```python
from build123d import *

# Parameters (mm, degrees)
F0_R           = 13.5
F0_R_2         = 10.75
F1_DEPTH       = 5
F2_R           = 25
F2_R_2         = 13.5
F2_R_3         = 10.75
F3_DEPTH       = 7
F4_R           = 17.5
F5_DEPTH       = 27
F6_R           = 30
F6_R_2         = 17.5
F7_DEPTH       = 11
F8_R           = 22.5
F9_DEPTH       = 49
F10_R          = 15
F11_DEPTH      = 4
F12_R          = 17
F12_R_2        = 15
F13_DEPTH      = 5
F14_R          = 11.5
F15_DEPTH      = 37
F16_R          = 10.75
F17_DEPTH      = 103.001
F18_SIZE       = 0.5
F19_SIZE2      = 2.99999
F19_SIZE       = 7.49999
F20_SIZE       = 0.5
F22_R          = 10
F23_DEPTH      = 57
F23_DEPTH_BACK = 11
F24_R          = 8
F25_DEPTH      = 71.2396442793
F26_R          = 17
F26_R_2        = 10
F26_R_3        = 8
F27_DEPTH      = 7
F28_SIZE2      = 6.99999
F28_SIZE       = 2.99999
F30_R          = 1.25
F33_R          = 11.5
F34_DEPTH      = 1.1


# Not quite as in the source:
# - a fillet or chamfer that OpenCascade refuses, or shapes differently, is made with other operations: its cross-section is extruded or revolved along the edge and cut away or added
# - a fillet or chamfer is up to 0.001 mm smaller than in the source, because OpenCascade refuses the exact size


with BuildPart() as f1:
    # F0 (on Top) → F1 (new body)
    with BuildSketch(Plane.XY):
        Circle(F0_R)
        Circle(F0_R_2, mode=Mode.SUBTRACT)
    extrude(amount=F1_DEPTH)

    # F2 (on face) → F3 (join)
    with BuildSketch(Plane(origin=(0, 0, 0), x_dir=(1, 0, 0), z_dir=(0, 0, -1))):
        Circle(F2_R)
        Circle(F2_R_2, mode=Mode.SUBTRACT)
        Circle(F2_R_2)
        Circle(F2_R_3, mode=Mode.SUBTRACT)
    extrude(amount=F3_DEPTH)

    # F4 (on face) → F5 (join)
    with BuildSketch(Plane(origin=(0, 0, -7), x_dir=(1, 0, 0), z_dir=(0, 0, -1))):
        Circle(F4_R)
    extrude(amount=F5_DEPTH)

    # F6 (on face) → F7 (join)
    with BuildSketch(Plane(origin=(0, 0, -34), x_dir=(1, 0, 0), z_dir=(0, 0, -1))):
        Circle(F6_R)
        Circle(F6_R_2, mode=Mode.SUBTRACT)
        Circle(F6_R_2)
    extrude(amount=F7_DEPTH)

    # F8 (on face) → F9 (join)
    with BuildSketch(Plane(origin=(0, 0, -45), x_dir=(1, 0, 0), z_dir=(0, 0, -1))):
        Circle(F8_R)
    extrude(amount=F9_DEPTH)

    # F10 (on face) → F11 (join)
    with BuildSketch(Plane(origin=(0, 0, -94), x_dir=(1, 0, 0), z_dir=(0, 0, -1))):
        Circle(F10_R)
    extrude(amount=F11_DEPTH)

    # F12 (on face) → F13 (join)
    with BuildSketch(Plane(origin=(0, 0, -98), x_dir=(1, 0, 0), z_dir=(0, 0, -1))):
        Circle(F12_R)
        Circle(F12_R_2, mode=Mode.SUBTRACT)
        Circle(F12_R_2)
    extrude(amount=F13_DEPTH)

    # F14 (on face) → F15 (cut)
    with BuildSketch(Plane(origin=(0, 0, -103), x_dir=(1, 0, 0), z_dir=(0, 0, -1))):
        Circle(F14_R)
    extrude(amount=-F15_DEPTH, mode=Mode.SUBTRACT)

    # F16 (on face) → F17 (cut, through all)
    with BuildSketch(Plane.XY):
        Circle(F16_R)
    extrude(amount=-F17_DEPTH, mode=Mode.SUBTRACT)

    # F18
    f18_edges = [f1.edges().sort_by_distance(p)[0] for p in [
        (-11.5, 0, -103),
        (-22.5, 0, -94),
        (-30, 0, -45),
        (-30, 0, -34),
        (-25, 0, 0),
        (-13.5, 0, 5),
        (-10.75, 0, 5),
    ]]
    chamfer(f18_edges, length=F18_SIZE)

    # F19 (size 7.5 and 3 in the source; OpenCascade refuses exactly that, so slightly less here)
    f19_edges = [f1.edges().sort_by_distance(p)[0] for p in [
        (-25, 0, -7),
    ]]
    f19_side = f1.faces().sort_by_distance((-24.292893, 0, -7))[0]
    chamfer(f19_edges, length=F19_SIZE, length2=F19_SIZE2, reference=f19_side)

    # F20
    f20_edges = [f1.edges().sort_by_distance(p)[0] for p in [
        (-25, 0, -4.00001),
    ]]
    chamfer(f20_edges, length=F20_SIZE)

    # F22 (on offset) → F23 (join, two sides)
    with BuildSketch(Plane.XZ.offset(22.5)) as f23_sk:
        with Locations((0, -79)):
            Circle(F22_R)
    extrude(amount=F23_DEPTH)
    extrude(f23_sk.sketch, amount=-F23_DEPTH_BACK)

    # F24 (on face) → F25 (cut, through all)
    with BuildSketch(Plane.XZ.offset(79.5)):
        with Locations((0, -79)):
            Circle(F24_R)
    extrude(amount=-F25_DEPTH, mode=Mode.SUBTRACT)

    # F26 (on face) → F27 (join)
    with BuildSketch(Plane.XZ.offset(79.5)):
        with Locations((0, -79)):
            Circle(F26_R)
        with Locations((0, -79)):
            Circle(F26_R_2, mode=Mode.SUBTRACT)
        with Locations((0, -79)):
            Circle(F26_R_2)
        with Locations((0, -79)):
            Circle(F26_R_3, mode=Mode.SUBTRACT)
    extrude(amount=F27_DEPTH)

    # F28 (size 3 and 7 in the source; OpenCascade refuses exactly that, so slightly less here)
    f28_edges = [f1.edges().sort_by_distance(p)[0] for p in [
        (-17, -79.5, -79),
    ]]
    f28_side = f1.faces().sort_by_distance((-17, -83, -79))[0]
    chamfer(f28_edges, length=F28_SIZE, length2=F28_SIZE2, reference=f28_side)

    # F29: chamfer of 0.5 on 2 edges, made by hand

    # F29_s1 → F29_t2 (revolve, cut)
    with BuildSketch(Plane.XY.offset(-79)):
        Polygon((17, -86), (16.5, -86.5), (17, -86.5), align=None)
    revolve(axis=Axis((0, -86.5, -79), (0, -1, 0)), mode=Mode.SUBTRACT)

    # F29_s3 → F29_t4 (revolve, cut)
    with BuildSketch(Plane.XY.offset(-79)):
        Polygon((16.6969593323, -82.3701156755), (17, -82.8296883264), (17, -82.49999), align=None)
    revolve(axis=Axis((0, -82.49999, -79), (0, -1, 0)), mode=Mode.SUBTRACT)

    # F30 (on Right) → F31 (revolve, cut)
    with BuildSketch(Plane.YZ):
        with Locations((-86.5, -66)):
            Circle(F30_R)
    revolve(axis=Axis((0, -66.6620582342, -79), (0, -1, 0)), mode=Mode.SUBTRACT)

    # F33 (on offset) → F34 (cut)
    with BuildSketch(Plane.XY.offset(1)):
        Circle(F33_R)
    extrude(amount=-F34_DEPTH, mode=Mode.SUBTRACT)


solid = f1.part
```
Check sheet for the modelled part. Datum: model origin and axes. Units: mm. A direction names the side the tool comes from. Give positions to 0.01 mm unless a question says otherwise; leave off trailing zeros. Write each loop counter-clockwise with the first axis right and the second up, starting at its lowest first coordinate (ties: lowest second). Pieces come first, ordered by that corner, then holes. Notation, with made-up numbers: (70, 25.5) - (98, 25.5) arc R23 cw to (98, 59.5) - close; hole circle Ø4 at (79.25, 84.5). An arc over 180 degrees is marked (long way). Answer as a JSON object with one key per item and string values. Group by question number.
1) Sectioned sample at B-B (x = 0). Give the number of separate pieces and of enclosed holes in the cut face, then the cut area to 3 significant figures.
2) Depth check by flat-ended pin: P1, Ø5, axis at y = -51.5, z = -73, coming from the +X side; P2, Ø11.5, axis at x = 5, y = 1, coming from the -Z side; P3, Ø1, axis at y = -44, z = -80.5, coming from the -X side; P4, Ø14, axis at x = 0, y = 0, coming from the +Z side. Enter the tip coordinate at first touch or a pass-through.
3) Access from +Z, -Z, +X, -X, +Y, -Y to the whole of each face (thin tool, end or side, straight path). Record for faces 1 (the face through (-2.493, 11.227, -84.506)), 2 (the face through (-1.34, -79.64, -68.76)), 3 (the face through (-1.4, 10.66, 2.77)), 4 (the face through (11, 11, 0)), 5 (the face through (-6, 10, 5)).
4) Sectioned sample at C-C (z = -48.5). Record the cut outline in (x, y), then the cut area to 3 significant figures.
5) Release check for a two-part mould opening along X. For faces 6 (the face through (-29.97, -1.32, -39.43)), 7 (the face through (-14, -86.5, -84)), 8 (the face through (8, -8, 1)) record: pulls with the +X half, pulls with the -X half, needs draft (parallel to the pull), parting line crosses it, or undercut.
6) Sectioned sample at D-D (y = -42). Record the cut outline in (x, z).
7) Thickness scan on probe 1 along Z at (x, y) = (0, -34.5); probe 2 along Z at (x, y) = (-12, 11); probe 3 along X at (y, z) = (0, -86). Record the ranges inside material, lowest first. Write a range as from..to.
Geometry results:
{
 "1": {"separate pieces": "3", "enclosed holes": "0", "area": "2,330 mm^2"},
 "2": {"P1": "stops at x = 9.37", "P2": "stops at z = -66", "P3": "stops at x = -9.95", "P4": "passes through"},
 "3": {"face 1": "-Z", "face 2": "none", "face 3": "+Z, -Z", "face 4": "+Z", "face 5": "+Z, +X, -X, +Y, -Y"},
 "4": {"outline": "circle Ø45 at (0, 0); hole circle Ø21.5 at (0, 0)", "area": "1,230 mm^2"},
 "5": {"face 6": "parting line crosses it", "face 7": "needs draft", "face 8": "undercut"},
 "6": {"outline": "circle Ø20 at (0, -79); hole circle Ø16 at (0, -79)"},
 "7": {"probe 1": "z = -89..-87, -71..-69", "probe 2": "z = -103..-98, -94..0", "probe 3": "x = -22.5..-11.5, 11.5..22.5"}
}
